Could you check a few things on this model? Use its own coordinates, in mm. Face numbers are marked on the shaded views. A direction names the side the tool comes from. Round coordinates to 2 decimals unless told otherwise and drop trailing zeros. Write each loop counter-clockwise with the first axis right and the second up, starting at its lowest first coordinate (ties: lowest second). Pieces come first, ordered by that corner, then holes. Notation, with made-up numbers: (-5.5, 48) -> (28.5, 48) arc R26 cw to (28.5, 86) -> close; hole circle Ø3 at (4.25, 35). An arc over 180 degrees is marked (long way). Return JSON: item names as keys, results as strings.
from build123d import *

# Parameters (mm, degrees)
SKIZZE1_W                                            = 65
SKIZZE1_H                                            = 65
AUFSATZ_LINEAR_AUSTRAGEN1_DEPTH                      = 14.5
STIRNSENKUNG_F_R_M6_ZYLINDERSCHRAUBE_MIT_D           = 6.6
STIRNSENKUNG_F_R_M6_ZYLINDERSCHRAUBE_MIT_CBORE_D     = 11
STIRNSENKUNG_F_R_M6_ZYLINDERSCHRAUBE_MIT_CBORE_DEPTH = 6.4
SKIZZE8_W                                            = 65
SKIZZE8_H                                            = 36
SCHNITT_LINEAR_AUSTRAGEN1_DEPTH                      = 2
KERNLOCH_F_R_M5_GEWINDE1_D                           = 4.2


with BuildPart() as part:
    # Skizze1 → Aufsatz-Linear austragen1 (new body)
    with BuildSketch(Plane(origin=(0, 0, 0), x_dir=(1, 0, 0), z_dir=(0, 1, 0))):
        Rectangle(SKIZZE1_W, SKIZZE1_H)
    extrude(amount=AUFSATZ_LINEAR_AUSTRAGEN1_DEPTH)

    # Stirnsenkung für M6 Zylinderschraube mit Innensechskant1 (through all)
    with Locations(Plane(origin=(0, 14.5, 0), x_dir=(1, 0, 0), z_dir=(0, 1, 0))):
        with Locations((-25, -25), (-25, 25), (25, 25), (25, -25)):
            CounterBoreHole(STIRNSENKUNG_F_R_M6_ZYLINDERSCHRAUBE_MIT_D / 2, STIRNSENKUNG_F_R_M6_ZYLINDERSCHRAUBE_MIT_CBORE_D / 2, STIRNSENKUNG_F_R_M6_ZYLINDERSCHRAUBE_MIT_CBORE_DEPTH)

    # Skizze8 → Schnitt-Linear austragen1 (cut)
    with BuildSketch(Plane(origin=(0, 14.5, 0), x_dir=(1, 0, 0), z_dir=(0, 1, 0))):
        with Locations((0, 0.5)):
            Rectangle(SKIZZE8_W, SKIZZE8_H)
    extrude(amount=-SCHNITT_LINEAR_AUSTRAGEN1_DEPTH, mode=Mode.SUBTRACT)

    # Kernloch für M5 Gewinde1 (through all)
    with Locations(Plane(origin=(61.744554923, 12.5, 78.125902763), x_dir=(0, 0, 1), z_dir=(0, 1, 0))):
        with Locations((-68.625902763, -37.244554923), (-87.625902763, -37.244554923), (-87.625902763, -86.244554923), (-68.625902763, -86.244554923)):
            Hole(KERNLOCH_F_R_M5_GEWINDE1_D / 2)


solid = part.part
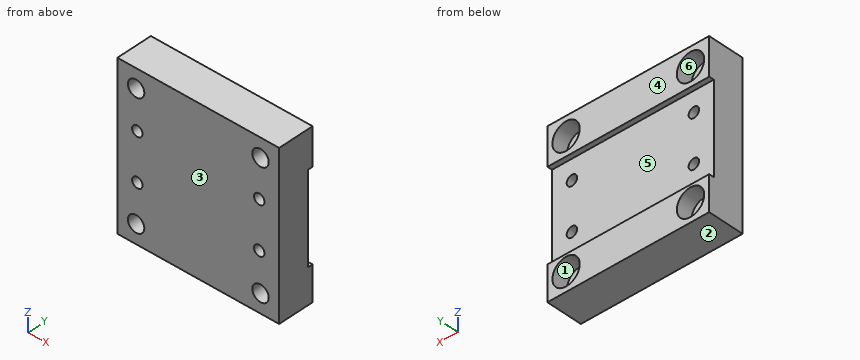
1) If I drill on probe 1 along X at (y, z) = (6.5, -9.5); probe 2 along X at (y, z) = (2.25, -25); probe 3 along Z at (x, y) = (-25, 11), over which ranges is the centre line in solid material (lowest first)? Write a range as [from, to].
Return value:
{"probe 1": "[-32.5, -26.6], [-22.4, 22.4], [26.6, 32.5]", "probe 2": "[-32.5, -28.3], [-21.7, 21.7], [28.3, 32.5]", "probe 3": "[-32.5, -30.5], [-19.5, -11.54], [-7.46, 7.46], [11.54, 19.5], [30.5, 32.5]"}
2) For the marked faces 4, 5 and 6, which set-ups out of +Z, -Z, +X, -X, +Y, -Y let a thin tool reach every point of the face, with its end or its side?
Return value:
{"face 4": "+Z, -Z, +X, -X, +Y", "face 5": "+X, -X, +Y", "face 6": "+Y"}
3) I want a section at D-D, the plane x = -24.5. Count the separate pieces of the cut face and the enclosed holes in it, and give its area (3 significant figures).
Return value:
{"separate pieces": "5", "enclosed holes": "0", "area": "520 mm²"}
4) Thinking about a two-plate mould opening in Z: for the marked faces 1, 2 and 3, which applies, pulls with the +Z half, pulls with the -Z half, needs draft (parallel to the pull), parting line crosses it, or undercut?
Return value:
{"face 1": "undercut", "face 2": "pulls with the -Z half", "face 3": "needs draft"}
5) I want a section at B-B, the plane x = -9. Please give me the cut outline in (y, z), and give its area (4 significant figures).
Return value:
{"outline": "(0, -32.5) -> (14.5, -32.5) -> (14.5, -18.5) -> (12.5, -18.5) -> (12.5, 17.5) -> (14.5, 17.5) -> (14.5, 32.5) -> (0, 32.5) -> close", "area": "870.5 mm²"}
6) Will these pins go through, and if not, where does the flat tip stop? pin 1 Ø7.5 at (x, z) = (25, -25) entering from +Y; pin 2 Ø5 at (x, z) = (24.5, -9.5) entering from +Y; pin 3 Ø6.5 at (x, z) = (-25, -25) entering from -Y.
Return value:
{"pin 1": "y = 8.1", "pin 2": "y = 12.5", "pin 3": "through"}
7) I want a section at C-C, the plane z = 9.5. Please give me the cut outline in (x, y).
Return value:
{"outline": "(-32.5, 0) -> (-26.6, 0) -> (-26.6, 12.5) -> (-32.5, 12.5) -> close; (-22.4, 0) -> (22.4, 0) -> (22.4, 12.5) -> (-22.4, 12.5) -> close; (26.6, 0) -> (32.5, 0) -> (32.5, 12.5) -> (26.6, 12.5) -> close"}
8) I want a section at A-A, the plane z = -25. Please give me the cut outline in (x, y).
Return value:
{"outline": "(-32.5, 0) -> (-28.3, 0) -> (-28.3, 8.1) -> (-30.5, 8.1) -> (-30.5, 14.5) -> (-32.5, 14.5) -> close; (-21.7, 0) -> (21.7, 0) -> (21.7, 8.1) -> (19.5, 8.1) -> (19.5, 14.5) -> (-19.5, 14.5) -> (-19.5, 8.1) -> (-21.7, 8.1) -> close; (28.3, 0) -> (32.5, 0) -> (32.5, 14.5) -> (30.5, 14.5) -> (30.5, 8.1) -> (28.3, 8.1) -> close"}
